from build123d import *

# Parameters (mm, degrees)
SKETCH1_R           = 1.95
BOSS_EXTRUDE1_DEPTH = 15
CUT_EXTRUDE2_DEPTH  = 16
CUT_EXTRUDE3_DEPTH  = 16
CUT_EXTRUDE4_DEPTH  = 16
CUT_EXTRUDE5_DEPTH  = 16
FILLET1_R           = 5
SKETCH7_W           = 220
SKETCH7_H           = 267.35226683
CUT_EXTRUDE6_DEPTH  = 11
CUT_EXTRUDE7_DEPTH  = 271.35226683
FILLET2_R           = 2.5


with BuildPart() as part:
    # Sketch1 → Boss-Extrude1 (new body)
    with BuildSketch(Plane(origin=(122, 0, 0), x_dir=(0, -1, 0), z_dir=(-1, 0, 0))):
        with BuildLine():
            Line((-67.5, -1.6625), (202.85226683, -1.6625))
            Line((202.85226683, -1.6625), (202.85226683, 220.3375))
            Line((202.85226683, 220.3375), (114.499999998, 220.3375))
            Line((114.499999998, 220.3375), (114.499999998, 108.985233168))
            ThreePointArc((114.499999998, 108.985233168), (102.08199146, 79.005508538), (72.10226683, 66.5875))
            Line((72.10226683, 66.5875), (-52.25, 66.5875))
            ThreePointArc((-52.25, 66.5875), (-63.033378413, 62.120878413), (-67.5, 51.3375))
            Line((-67.5, 51.3375), (-67.5, -1.6625))
        make_face()
        with Locations((-60.5, 6.5875)):
            Circle(SKETCH1_R, mode=Mode.SUBTRACT)
        with Locations((107.5, 6.5875)):
            Circle(SKETCH1_R, mode=Mode.SUBTRACT)
        with Locations((-60.5, 45.5875)):
            Circle(SKETCH1_R, mode=Mode.SUBTRACT)
        with Locations((-46.5, 59.5875)):
            Circle(SKETCH1_R, mode=Mode.SUBTRACT)
        with Locations((45.5, 59.5875)):
            Circle(SKETCH1_R, mode=Mode.SUBTRACT)
        Polygon((42.95, 15.7375), (42.95, 13.2375), (40.95, 11.3375), (33.95, 11.3375), (31.95, 13.2375), (31.95, 15.7375), align=None, mode=Mode.SUBTRACT)
        with BuildLine():
            Line((30.95, 11.3375), (17.5, 11.3375))
            Line((17.5, 11.3375), (17.5, 13.9375))
            ThreePointArc((17.5, 13.9375), (24.225, 16.3375), (30.95, 13.9375))
            Line((30.95, 13.9375), (30.95, 11.3375))
        make_face(mode=Mode.SUBTRACT)
    extrude(amount=-BOSS_EXTRUDE1_DEPTH)

    # Sketch2 → Cut-Extrude2 (cut, through all)
    with BuildSketch(Plane(origin=(137, 0, 0), x_dir=(0, 0, -1), z_dir=(1, 0, 0))):
        with BuildLine():
            Line((-42.5875, 53.5), (-13.3375, 53.5))
            ThreePointArc((-13.3375, 53.5), (-6.266432188, 50.571067812), (-3.3375, 43.5))
            Line((-3.3375, 43.5), (-3.3375, 16))
            ThreePointArc((-3.3375, 16), (-6.266432188, 8.928932188), (-13.3375, 6))
            Line((-13.3375, 6), (-42.5875, 6))
            ThreePointArc((-42.5875, 6), (-49.658567812, 8.928932188), (-52.5875, 16))
            Line((-52.5875, 16), (-52.5875, 43.5))
            ThreePointArc((-52.5875, 43.5), (-49.658567812, 50.571067812), (-42.5875, 53.5))
        make_face()
        with BuildLine():
            Line((-42.5875, -46.5), (-15.3375, -46.5))
            ThreePointArc((-15.3375, -46.5), (-8.266432188, -43.571067812), (-5.3375, -36.5))
            Line((-5.3375, -36.5), (-5.3375, -9))
            ThreePointArc((-5.3375, -9), (-8.266432188, -1.928932188), (-15.3375, 1))
            Line((-15.3375, 1), (-42.5875, 1))
            ThreePointArc((-42.5875, 1), (-49.658567812, -1.928932188), (-52.5875, -9))
            Line((-52.5875, -9), (-52.5875, -36.5))
            ThreePointArc((-52.5875, -36.5), (-49.658567812, -43.571067812), (-42.5875, -46.5))
        make_face()
        with BuildLine():
            Line((-55.22929809, -61.015037849), (-16.864289826, -103.641109909))
            ThreePointArc((-16.864289826, -103.641109909), (-16.438731405, -106.33063253), (-18.722491736, -107.81355891))
            Line((-18.722491736, -107.81355891), (-54.5875, -107.81355891))
            ThreePointArc((-54.5875, -107.81355891), (-58.123033906, -106.349092816), (-59.5875, -102.81355891))
            Line((-59.5875, -102.81355891), (-59.5875, -62.68748685))
            ThreePointArc((-59.5875, -62.68748685), (-57.983182763, -60.353444779), (-55.22929809, -61.015037849))
        make_face()
        with BuildLine():
            Line((-44.725753318, -51.5), (-15.3375, -51.5))
            ThreePointArc((-15.3375, -51.5), (-8.266432188, -54.428932188), (-5.3375, -61.5))
            Line((-5.3375, -61.5), (-5.3375, -94.985299242))
            ThreePointArc((-5.3375, -94.985299242), (-6.941817237, -97.319341313), (-9.69570191, -96.657748243))
            Line((-9.69570191, -96.657748243), (-46.583955228, -55.672449001))
            ThreePointArc((-46.583955228, -55.672449001), (-47.00951365, -52.98292638), (-44.725753318, -51.5))
        make_face()
    extrude(amount=-CUT_EXTRUDE2_DEPTH, mode=Mode.SUBTRACT)

    # Sketch3 → Cut-Extrude3 (cut, through all)
    with BuildSketch(Plane(origin=(137, 0, 0), x_dir=(0, 0, -1), z_dir=(1, 0, 0))):
        with BuildLine():
            Line((-212.5875, -129.499999998), (-108.985233168, -129.499999998))
            ThreePointArc((-108.985233168, -129.499999998), (-106.235233168, -132.249999998), (-108.985233168, -134.999999998))
            Line((-108.985233168, -134.999999998), (-212.5875, -134.999999998))
            ThreePointArc((-212.5875, -134.999999998), (-215.3375, -132.249999998), (-212.5875, -129.499999998))
        make_face()
        with BuildLine():
            Line((-212.5875, -179.499999998), (-108.985233168, -179.499999998))
            ThreePointArc((-108.985233168, -179.499999998), (-106.235233168, -182.249999998), (-108.985233168, -184.999999998))
            Line((-108.985233168, -184.999999998), (-212.5875, -184.999999998))
            ThreePointArc((-212.5875, -184.999999998), (-215.3375, -182.249999998), (-212.5875, -179.499999998))
        make_face()
    extrude(amount=-CUT_EXTRUDE3_DEPTH, mode=Mode.SUBTRACT)

    # Sketch4 → Cut-Extrude4 (cut, through all)
    with BuildSketch(Plane(origin=(137, 0, 0), x_dir=(0, 0, -1), z_dir=(1, 0, 0))):
        with BuildLine():
            Line((-94.235233168, -187.642635713), (-94.235233168, -135.242622679))
            ThreePointArc((-94.235233168, -135.242622679), (-92.796770819, -132.97918772), (-90.136722915, -133.320445536))
            Line((-90.136722915, -133.320445536), (-24.120536911, -188.22045857))
            ThreePointArc((-24.120536911, -188.22045857), (-23.367936485, -190.992505451), (-25.719047164, -192.642635713))
            Line((-25.719047164, -192.642635713), (-89.235233168, -192.642635713))
            ThreePointArc((-89.235233168, -192.642635713), (-92.770767074, -191.178169619), (-94.235233168, -187.642635713))
        make_face()
        with BuildLine():
            Line((-12.547131117, -129.709631116), (-12.547131117, -182.109644149))
            ThreePointArc((-12.547131117, -182.109644149), (-13.985593467, -184.373079109), (-16.64564137, -184.031821292))
            Line((-16.64564137, -184.031821292), (-82.661827375, -129.131808259))
            ThreePointArc((-82.661827375, -129.131808259), (-83.414427801, -126.359761378), (-81.063317121, -124.709631116))
            Line((-81.063317121, -124.709631116), (-17.547131117, -124.709631116))
            ThreePointArc((-17.547131117, -124.709631116), (-14.011597211, -126.17409721), (-12.547131117, -129.709631116))
        make_face()
    extrude(amount=-CUT_EXTRUDE4_DEPTH, mode=Mode.SUBTRACT)

    # Sketch5 → Cut-Extrude5 (cut, through all)
    with BuildSketch(Plane(origin=(137, 0, 0), x_dir=(0, 0, -1), z_dir=(1, 0, 0))):
        with BuildLine():
            Line((-210.3375, -146.999999998), (-210.3375, -167.499999998))
            ThreePointArc((-210.3375, -167.499999998), (-208.873033906, -171.035533904), (-205.3375, -172.499999998))
            Line((-205.3375, -172.499999998), (-183.830323645, -172.499999998))
            ThreePointArc((-183.830323645, -172.499999998), (-180.294789739, -171.035533904), (-178.830323645, -167.499999998))
            Line((-178.830323645, -167.499999998), (-178.830323645, -146.999999998))
            ThreePointArc((-178.830323645, -146.999999998), (-180.294789739, -143.464466093), (-183.830323645, -141.999999998))
            Line((-183.830323645, -141.999999998), (-205.3375, -141.999999998))
            ThreePointArc((-205.3375, -141.999999998), (-208.873033906, -143.464466093), (-210.3375, -146.999999998))
        make_face()
        with BuildLine():
            Line((-173.830323645, -146.999999998), (-173.830323645, -167.499999998))
            ThreePointArc((-173.830323645, -167.499999998), (-172.365857551, -171.035533904), (-168.830323645, -172.499999998))
            Line((-168.830323645, -172.499999998), (-147.323147289, -172.499999998))
            ThreePointArc((-147.323147289, -172.499999998), (-143.787613384, -171.035533904), (-142.323147289, -167.499999998))
            Line((-142.323147289, -167.499999998), (-142.323147289, -146.999999998))
            ThreePointArc((-142.323147289, -146.999999998), (-143.787613384, -143.464466093), (-147.323147289, -141.999999998))
            Line((-147.323147289, -141.999999998), (-168.830323645, -141.999999998))
            ThreePointArc((-168.830323645, -141.999999998), (-172.365857551, -143.464466093), (-173.830323645, -146.999999998))
        make_face()
        with BuildLine():
            Line((-137.323147289, -146.999999998), (-137.323147289, -167.499999998))
            ThreePointArc((-137.323147289, -167.499999998), (-135.858681195, -171.035533904), (-132.323147289, -172.499999998))
            Line((-132.323147289, -172.499999998), (-110.815970934, -172.499999998))
            ThreePointArc((-110.815970934, -172.499999998), (-107.280437028, -171.035533904), (-105.815970934, -167.499999998))
            Line((-105.815970934, -167.499999998), (-105.815970934, -146.999999998))
            ThreePointArc((-105.815970934, -146.999999998), (-107.280437028, -143.464466093), (-110.815970934, -141.999999998))
            Line((-110.815970934, -141.999999998), (-132.323147289, -141.999999998))
            ThreePointArc((-132.323147289, -141.999999998), (-135.858681195, -143.464466093), (-137.323147289, -146.999999998))
        make_face()
    extrude(amount=-CUT_EXTRUDE5_DEPTH, mode=Mode.SUBTRACT)

    # Fillet1
    fillet1_edges = [part.edges().sort_by_distance(p)[0] for p in [
        (129.5, -114.499999998, 220.3375),
        (129.5, -202.85226683, 220.3375),
    ]]
    fillet(fillet1_edges, radius=FILLET1_R)

    # Sketch7 → Cut-Extrude6 (cut)
    with BuildSketch(Plane(origin=(137, 0, 0), x_dir=(0, 0, -1), z_dir=(1, 0, 0))):
        with Locations((-110.3375, -67.676133415)):
            Rectangle(SKETCH7_W, SKETCH7_H)
    extrude(amount=-CUT_EXTRUDE6_DEPTH, mode=Mode.SUBTRACT)

    # Sketch8 → Cut-Extrude7 (cut, through all)
    with BuildSketch(Plane.XZ.offset(202.85226683)):
        Polygon((137, 54.353248627), (137, 242.443718096), (126, 242.443718096), (126, 38.3375), (137, 8.3375), align=None)
    extrude(amount=-CUT_EXTRUDE7_DEPTH, mode=Mode.SUBTRACT)

    # Fillet2
    fillet2_edges = [part.edges().sort_by_distance(p)[0] for p in [
        (131.5, 66, 0.3375),
        (131.5, -201.35226683, 0.3375),
    ]]
    fillet(fillet2_edges, radius=FILLET2_R)


solid = part.part
CAD build for the part. Positions are in the model's coordinates, mm. A direction names the side the tool comes from. Round coordinates to 2 decimals unless told otherwise and drop trailing zeros. Order: outer loops, then holes, each group sorted by start corner. A loop starts at its lowest first (then second) coordinate and runs counter-clockwise, first axis right, second up. Notation, with made-up numbers: M 53.5,23.25 L 87.5,23.25 A24 ccw 87.5,39.25 Z; hole C -26.5,66.5 d2. An arc over 180 degrees is marked long. Use one line per item in the form item = value.
Q1. Probe L1, parallel to Y at x = 123.75, z = 196; L2, parallel to Z at x = 124.5, y = -174.5; L3, parallel to Z at x = 124.55, y = 60.5. List the from-to ranges inside material, lowest first.
Recorded:
L1 = -202.85 to -185, -179.5 to -172.5, -142 to -135, -129.5 to -114.5
L2 = -1.66 to 12.55, 28.11 to 40.62, 94.24 to 220.34
L3 = -1.66 to 4.64, 8.54 to 43.64, 47.54 to 64.16
Q2. Two-plate mould, pull along X, no slides. Class faces 4 (the flat face through (122, -117, 93)), 5 (the flat face through (125, -202.852, 82)), 6 (the flat face through (131.42, 66.74, 23.55)): +X half, -X half, draft (parallel to the pull), parting line (faces both ways), or undercut.
Recorded:
face_4 = -X half
face_5 = draft
face_6 = +X half
Q3. Which spindle directions (+Z, -Z, +X, -X, +Y, -Y) get a long thin tool onto all of the face, cutting with end or side? Do faces 1 (the flat face through (130, 66, 13)), 2 (the cylindrical face through (123.972, 62.914, 62.239)), 3 (the cylindrical face through (124.03, -43.49, 49.74)). Say none if no direction does.
Recorded:
face_1 = +Z, +X
face_2 = +Z, +X, -X, +Y
face_3 = +X, -X
Q4. Saw through at C-C on y = -152. Give the cut face in (x, z), then the cut area to 3 significant figures.
Recorded:
outline = M 122,-1.66 L 137,-1.66 L 137,0.34 L 126,0.34 L 126,12.55 L 122,12.55 Z; M 122,55.16 L 126,55.16 L 126,67.67 L 122,67.67 Z; M 122,94.24 L 126,94.24 L 126,105.82 L 122,105.82 Z; M 122,137.32 L 126,137.32 L 126,142.32 L 122,142.32 Z; M 122,173.83 L 126,173.83 L 126,178.83 L 122,178.83 Z; M 122,210.34 L 126,210.34 L 126,220.34 L 122,220.34 Z
area = 255 mm^2
Q5. Saw through at D-D on y = -90.5. Give the cut face in (x, z), then the cut area to 3 significant figures.
Recorded:
outline = M 122,-1.66 L 137,-1.66 L 137,0.34 L 126,0.34 L 126,5.34 L 122,5.34 Z; M 122,15.24 L 126,15.24 L 126,28.69 L 122,28.69 Z; M 122,59.59 L 126,59.59 L 126,70.79 L 122,70.79 Z
area = 149 mm^2
Q6. Saw through at B-B on z = 200. Give the cut face in (x, y).
Recorded:
outline = M 122,-202.85 L 126,-202.85 L 126,-185 L 122,-185 Z; M 122,-179.5 L 126,-179.5 L 126,-172.5 L 122,-172.5 Z; M 122,-142 L 126,-142 L 126,-135 L 122,-135 Z; M 122,-129.5 L 126,-129.5 L 126,-114.5 L 122,-114.5 Z
Q7. Flat gauge pins, fed straight in: P1, Ø1, axis at x = 132.5, y = -101.5, coming from the +Z side; P2, Ø4.5, axis at y = 46.5, z = 59.59, coming from the +X side; P3, Ø2, axis at x = 123.5, z = 59.5, coming from the +Y side. Where does each tip first touch, or does it go through?
Recorded:
P1 = 0.34
P2 = 126
P3 = 65.71
Q8. Saw through at A-A on y = -20.5. Give the cut face in (x, z).
Recorded:
outline = M 122,-1.66 L 137,-1.66 L 137,0.34 L 126,0.34 L 126,5.34 L 122,5.34 Z; M 122,52.59 L 126,52.59 L 126,66.59 L 122,66.59 Z
